```python
from build123d import *

# Parameters (mm, degrees)
SKETCH2_R           = 6.5
BOSS_EXTRUDE1_DEPTH = 2
BOSS_EXTRUDE2_DEPTH = 1.84
CHAMFER1_SIZE       = 0.25
CHAMFER2_SIZE       = 0.5


with BuildPart() as part:
    # Sketch1 → Revolve1 (revolve)
    with BuildSketch(Plane(origin=(0, 0, 0), x_dir=(1, 0, 0), z_dir=(0, 1, 0))):
        Polygon((0, 0), (12.4079, 0), (12.4079, 4.8), (13.4079, 4.8), (13.4079, 6.64), (0, 6.64), align=None)
    revolve(axis=Axis((0, 0, 0), (0, 0, -1)))

    # Sketch2 → Boss-Extrude1 (add)
    with BuildSketch(Plane.XY):
        Circle(SKETCH2_R)
    extrude(amount=BOSS_EXTRUDE1_DEPTH)

    # Sketch3 → Boss-Extrude2 (add)
    with BuildSketch(Plane(origin=(0, 0, -6.64), x_dir=(-1, 0, 0), z_dir=(0, 0, -1))):
        with BuildLine():
            Line((-21.81085625, -3.283793483), (-6.47460787, -11.741006572))
            ThreePointArc((-6.47460787, -11.741006572), (-13.4079, 0), (-6.474607871, 11.741006572))
            Line((-6.474607871, 11.741006572), (-21.81085625, 3.283793483))
            ThreePointArc((-21.81085625, 3.283793483), (-23.75, 0), (-21.81085625, -3.283793483))
        make_face()
    boss_extrude2 = extrude(amount=-BOSS_EXTRUDE2_DEPTH)

    # Sketch4 → #4 Clearance Hole1 (revolve, cut)
    with BuildSketch(Plane(origin=(20, 0, -6.64), x_dir=(0, 1, 0), z_dir=(1, 0, 0))):
        Polygon((0, 0), (0, 16.037806461), (1.7272, 15), (1.7272, 0), align=None)
    f_4_clearance_hole1 = revolve(axis=Axis((20, 0, -12.99), (0, 0, 1)), mode=Mode.SUBTRACT)

    # Mirror1: Boss-Extrude2, #4 Clearance Hole1 across plane
    add(boss_extrude2.mirror(Plane(origin=(0, 0, 0), x_dir=(0, 0, 1), z_dir=(1, 0, 0))))
    add(f_4_clearance_hole1.mirror(Plane(origin=(0, 0, 0), x_dir=(0, 0, 1), z_dir=(1, 0, 0))), mode=Mode.SUBTRACT)

    # Sketch8 → 1/16 NPT Tapped Hole2 (revolve, cut)
    with BuildSketch(Plane(origin=(0, 0, -6.64), x_dir=(0, 1, 0), z_dir=(1, 0, 0))):
        Polygon((0, 0), (0, 8.64), (3.0734, 8.64), (3.0734, 6.89), (3.781593923, 6.89), (3.968877, 0.635), (4.603877, 0), align=None)
    revolve(axis=Axis((0, 0, -12.99), (0, 0, 1)), mode=Mode.SUBTRACT)

    # Chamfer1
    chamfer1_edges = [part.edges().sort_by_distance(p)[0] for p in [
        (-12.4079, 0, 0),
    ]]
    chamfer(chamfer1_edges, length=CHAMFER1_SIZE)

    # Chamfer2
    chamfer2_edges = [part.edges().sort_by_distance(p)[0] for p in [
        (23.75, 0, -6.64),
        (14.14273206, -7.512400028, -6.64),
        (14.14273206, 7.512400028, -6.64),
        (0, -13.4079, -6.64),
        (-23.75, 0, -6.64),
        (-14.14273206, -7.512400028, -6.64),
        (-14.14273206, 7.512400028, -6.64),
        (0, 13.4079, -6.64),
    ]]
    chamfer(chamfer2_edges, length=CHAMFER2_SIZE)


solid = part.part
```
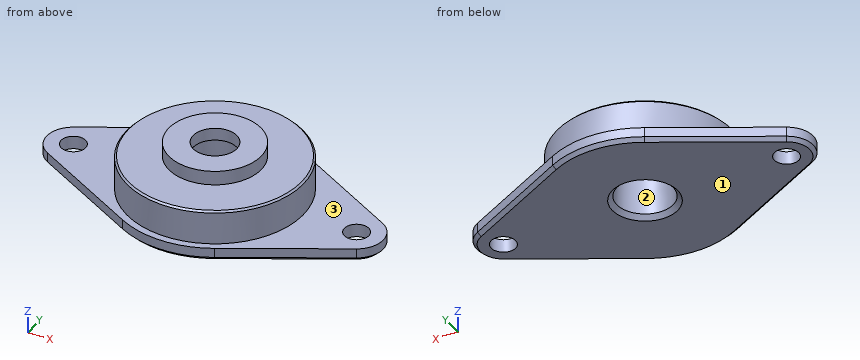
Part model, mm, in its own coordinate system. Face numbers are marked on the shaded views. A direction names the side the tool comes from. Round coordinates to 2 decimals unless told otherwise and drop trailing zeros. Loops run counter-clockwise (first coordinate to the right, second up) from the corner with the lowest first, then second, coordinate; pieces in that order, holes last.
1. Slice it at B-B (y = 0). Count the separate pieces of the cut face and the enclosed holes in it, and give its area (3 significant figures).
Solutions:
separate pieces: 4
enclosed holes: 0
area: 155 mm2
2. 3-axis set-ups, long thin cutter, end or side, ignore diameter. For the marked faces 1, 2 and 3: which of +Z, -Z, +X, -X, +Y, -Y reach the whole face in a straight line?
Solutions:
face 1: -Z, +X, -X, +Y, -Y
face 2: -Z
face 3: +Z
3. Slice it at C-C (z = -3.75). Give the cut face in (x, y).
Solutions:
outline: circle Ø24.82 at (0, 0); hole circle Ø7.8 at (0, 0)
4. Slice it at A-A (x = 0). Give the cut face in (y, z) (3 decimals), and give its area (3 significant figures).
Solutions:
outline: (-13.408, -6.14) - (-12.908, -6.64) - (-4.604, -6.64) - (-3.969, -6.005) - (-3.782, 0.25) - (-3.073, 0.25) - (-3.073, 2) - (-6.5, 2) - (-6.5, 0) - (-12.158, 0) - (-12.408, -0.25) - (-12.408, -4.8) - (-13.408, -4.8) - close; (3.073, 0.25) - (3.782, 0.25) - (3.969, -6.005) - (4.604, -6.64) - (12.908, -6.64) - (13.408, -6.14) - (13.408, -4.8) - (12.408, -4.8) - (12.408, -0.25) - (12.158, 0) - (6.5, 0) - (6.5, 2) - (3.073, 2) - close
area: 129 mm2
5. Drill centre lines: line 1 along Z through (x, y) = (-10, -4); line 2 along Z through (x, y) = (-11.5, -6.25); line 3 along Y through (x, z) = (20, -6.25). Where is each one in solid material? Low to high.
Solutions:
line 1: z = -6.64 to 0
line 2: z = -6.64 to -4.8
line 3: y = -4.16 to -1.73, 1.73 to 4.16
6. Flat gauge pins, fed straight in: pin 1 (5 mm diameter, centred on x = -4, z = -5.5, fed in from +Y); pin 2 (2 mm diameter, centred on x = 7.5, z = -1.5, fed in from +Y); pin 3 (3 mm diameter, centred on x = 5, z = -2.5, fed in from +Y). Where does each tip first touch, or does it go through?
Solutions:
pin 1: stops at y = 13.32
pin 2: stops at y = 10.57
pin 3: stops at y = 11.9
7. Slice it at D-D (x = -17.5). Give the cut face in (y, z).
Solutions:
outline: (-5.66, -6.14) - (-5.09, -6.64) - (5.09, -6.64) - (5.66, -6.14) - (5.66, -4.8) - (-5.66, -4.8) - close
